Design review of the part shown in the three views and the two pictorial views. Dimensions are in mm from the part's minimum x, y and z. Give positions to 0.01 mm unless a question says otherwise; leave off trailing zeros. Order: outer loops, then holes, each group sorted by start corner. A loop starts at its lowest first (then second) coordinate and runs counter-clockwise, first axis right, second up.
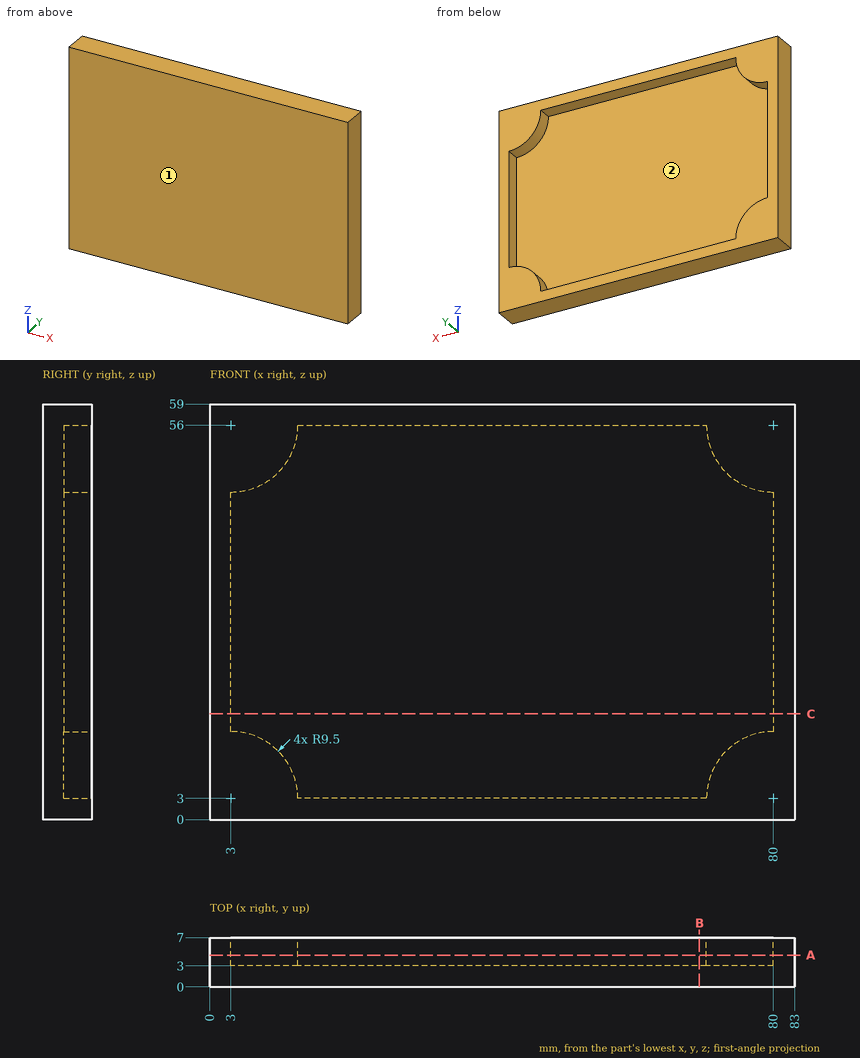
Item 1: Take a section at B-B (x = 69.5). Give the boundary of the cut face in (y, z), and give its area (3 significant figures).
Values found:
outline: (0, 0) - (7, 0) - (7, 3) - (3, 3) - (3, 56) - (7, 56) - (7, 59) - (0, 59) - close
area: 201 mm2
Item 2: For line 1 (X direction, y = 3.75, z = 41); line 2 (Z direction, x = 60, y = 6.5); line 3 (Y direction, x = 50.5, z = 11.5), list the stretches that pass through material, from the lowest coordinate up.
Values found:
line 1: x = 0 to 3, 80 to 83
line 2: z = 0 to 3, 56 to 59
line 3: y = 0 to 3
Item 3: Take a section at A-A (y = 4.5). Give the boundary of the cut face in (x, z).
Values found:
outline: (0, 0) - (83, 0) - (83, 59) - (0, 59) - close; hole (3, 12.5) arc R9.5 cw to (12.5, 3) - (70.5, 3) arc R9.5 cw to (80, 12.5) - (80, 46.5) arc R9.5 cw to (70.5, 56) - (12.5, 56) arc R9.5 cw to (3, 46.5) - close
Item 4: Draft analysis for pull direction X (two halves, no side actions). For the marked faces 1 and 2, state which applies: released by +X, released by -X, zero draft, split by the parting line, or undercut.
Values found:
face 1: zero draft
face 2: undercut
Item 5: Take a section at C-C (z = 15). Give the boundary of the cut face in (x, y), and give its area (3 significant figures).
Values found:
outline: (0, 0) - (83, 0) - (83, 7) - (80, 7) - (80, 3) - (3, 3) - (3, 7) - (0, 7) - close
area: 273 mm2
